Verification items for the finished model (mm, model axes). A direction names the side the tool comes from. Give positions to 0.01 mm unless a question says otherwise; leave off trailing zeros. Loops run counter-clockwise (first coordinate to the right, second up) from the corner with the lowest first, then second, coordinate; pieces in that order, holes last. Notation, with made-up numbers: (46, 51.25) - (80, 51.25) arc R15 ccw to (80, 79.25) - close; hole circle Ø4 at (10.5, -17.5). An arc over 180 degrees is marked (long way). Answer in a Markdown table with one row per item.
```python
from build123d import *

# Parameters (mm, degrees)
F0_W      = 19
F0_H      = 105
F1_DEPTH  = 5
F2_R      = 7.5
F3_DEPTH  = 5
F6_R      = 4.5
F7_DEPTH  = 10.001
F8_W      = 19
F8_H      = 30
F9_DEPTH  = 10
F10_R     = 4.5
F11_DEPTH = 11.001
F12_W     = 4
F12_H     = 20
F13_DEPTH = 5


with BuildPart() as f1:
    # F0 (on Front) → F1 (new body)
    with BuildSketch(Plane.XZ):
        with Locations((0, -42.5)):
            Rectangle(F0_W, F0_H)
    extrude(amount=F1_DEPTH)

    # F2 (on face) → F3 (join)
    with BuildSketch(Plane.XZ.offset(5)):
        Circle(F2_R)
    extrude(amount=F3_DEPTH)

    # F4 (on Right) → F5 (revolve)
    with BuildSketch(Plane.YZ):
        Polygon((-10, 5.5), (-10, 7.5), (-11, 7), (-11, 6), align=None)
    revolve(axis=Axis((0, -10.5, 0), (0, 1, 0)))

    # F6 (on face) → F7 (cut, through all)
    with BuildSketch(Plane.XZ.offset(10)):
        Circle(F6_R)
    extrude(amount=-F7_DEPTH, mode=Mode.SUBTRACT)

    # F8 (on face) → F9 (join)
    with BuildSketch(Plane(origin=(0, 0, 0), x_dir=(-1, 0, 0), z_dir=(0, 1, 0))):
        with Locations((0, -80)):
            Rectangle(F8_W, F8_H)
    extrude(amount=-F9_DEPTH)

    # F10 (on face) → F11 (cut, through all)
    with BuildSketch(Plane.XZ):
        with Locations((0, -80)):
            Circle(F10_R)
    extrude(amount=F11_DEPTH, mode=Mode.SUBTRACT)

    # F12 (on face) → F13 (cut, through all)
    with BuildSketch(Plane.XZ.offset(5)):
        with Locations((0, -17.5)):
            Rectangle(F12_W, F12_H)
    extrude(amount=-F13_DEPTH, mode=Mode.SUBTRACT)


solid = f1.part
```
Q1. Sectioned sample at A-A (y = -8.5). Record the cut outline in (x, z).
Completed:
| item | result |
|---|---|
| outline | (-9.5, -95) - (9.5, -95) - (9.5, -65) - (-9.5, -65) - close; circle Ø15 at (0, 0); hole circle Ø9 at (0, -80); hole circle Ø9 at (0, 0) |
Q2. Tool access check on faces 5 (the face through (0, -3, -27.5)), 6 (the face through (-5, -10, 0)), 7 (the face through (4, -10, -76)). Record the directions out of +Z, -Z, +X, -X, +Y, -Y that give a thin tool (end or side, any length) a straight path to the whole face; none if there is none.
Completed:
| item | result |
|---|---|
| face 5 | +Y, -Y |
| face 6 | -Y |
| face 7 | -Z, +X, -X, -Y |
Q3. Go/stop test with flat-tipped pins: P1, Ø6, axis at x = -1.5, z = -64, coming from the -Y side; P2, Ø5.5, axis at x = -1.5, z = -12, coming from the -Y side. Record where each tip stops, or that it passes through.
Completed:
| item | result |
|---|---|
| P1 | y = -10 |
| P2 | y = -5 |
Q4. Thickness scan on line 1 (Z direction, x = 0, y = -2.75); line 2 (Z direction, x = 0, y = -5.25); line 3 (Z direction, x = 4, y = -4). Record the ranges inside material, lowest first.
Completed:
| item | result |
|---|---|
| line 1 | -95 to -84.5, -75.5 to -27.5, -7.5 to -4.5, 4.5 to 10 |
| line 2 | -95 to -84.5, -75.5 to -65, -7.5 to -4.5, 4.5 to 7.5 |
| line 3 | -95 to -82.06, -77.94 to -2.06, 2.06 to 10 |
Q5. Sectioned sample at D-D (z = 0). Record the cut outline in (x, y), and give its area (3 significant figures).
Completed:
| item | result |
|---|---|
| outline | (-9.5, -5) - (-7.5, -5) - (-7.5, -10) - (-7, -11) - (-6, -11) - (-5.5, -10) - (-4.5, -10) - (-4.5, 0) - (-9.5, 0) - close; (4.5, -10) - (5.5, -10) - (6, -11) - (7, -11) - (7.5, -10) - (7.5, -5) - (9.5, -5) - (9.5, 0) - (4.5, 0) - close |
| area | 83.0 mm^2 |
Q6. Draft check along X on faces 1 (the face through (9.5, -4, -55)), 2 (the face through (2, -3, -18)), 3 (the face through (2, -11, 6)), 4 (the face through (-9.5, -4, -55)). Enter one of: +X half, -X half, draft (parallel to the pull), parting line (faces both ways), or undercut.
Completed:
| item | result |
|---|---|
| face 1 | +X half |
| face 2 | undercut |
| face 3 | draft |
| face 4 | -X half |
Q7. Sectioned sample at C-C (y = -2). Record the cut outline in (x, z).
Completed:
| item | result |
|---|---|
| outline | (-9.5, -95) - (9.5, -95) - (9.5, 10) - (-9.5, 10) - close; hole circle Ø9 at (0, -80); hole circle Ø9 at (0, 0); hole (-2, -27.5) - (2, -27.5) - (2, -7.5) - (-2, -7.5) - close |
Q8. Sectioned sample at B-B (z = -80). Record the cut outline in (x, y).
Completed:
| item | result |
|---|---|
| outline | (-9.5, -10) - (-4.5, -10) - (-4.5, 0) - (-9.5, 0) - close; (4.5, -10) - (9.5, -10) - (9.5, 0) - (4.5, 0) - close |
